The model under review builds one solid part; all positions refer to its coordinate system, in mm. Face numbers are marked on the shaded views. Coordinates: 2 decimals unless noted, no trailing zeros. Order: outer loops, then holes, each group sorted by start corner. A loop starts at its lowest first (then second) coordinate and runs counter-clockwise, first axis right, second up. Notation, with made-up numbers: (12, 87.25) - (26, 87.25) arc R25 cw to (26, 126.25) - close; hole circle Ø6 at (60.5, 69.5). An arc over 180 degrees is marked (long way). Answer in a Markdown table with one row per item.
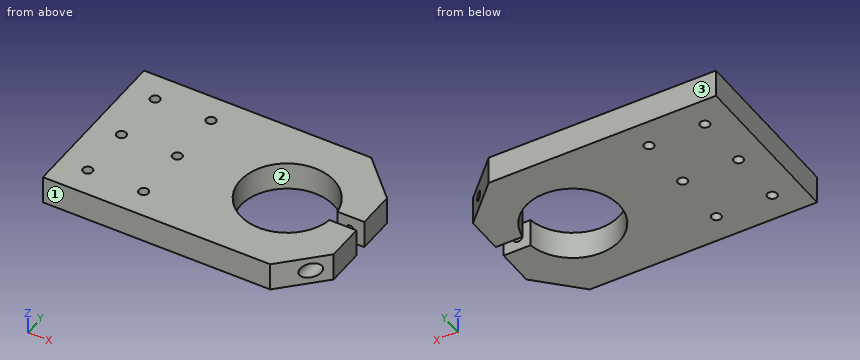
```python
from build123d import *

# Parameters (mm, degrees)
F0_R     = 2.182812
F0_R_2   = 2.182813
F1_DEPTH = 6.35
F2_R     = 3.5
F2_R_2   = 2.182813
F3_DEPTH = 25
F2_R_3   = 1.785938
F4_DEPTH = 35.1
F5_DEPTH = 76.2


with BuildPart() as f1:
    # F0 (on Top) → F1 (new body, symmetric)
    with BuildSketch(Plane.XY):
        with BuildLine():
            ThreePointArc((21.037169, -3), (-21.25, 0), (21.037169, 3))
            Line((21.037169, 3), (33.25, 3))
            Line((33.25, 3), (33.25, 20.1))
            Line((33.25, 20.1), (15.25, 38.1))
            Line((15.25, 38.1), (-88.05, 38.1))
            Line((-88.05, 38.1), (-88.05, -38.1))
            Line((-88.05, -38.1), (15.25, -38.1))
            Line((15.25, -38.1), (33.25, -20.1))
            Line((33.25, -20.1), (33.25, -3))
            Line((33.25, -3), (21.037169, -3))
        make_face()
        with Locations((-75.35, -25.4)):
            Circle(F0_R, mode=Mode.SUBTRACT)
        with Locations((-49.95, -25.4)):
            Circle(F0_R_2, mode=Mode.SUBTRACT)
        with Locations((-75.35, 0)):
            Circle(F0_R, mode=Mode.SUBTRACT)
        with Locations((-49.95, 0)):
            Circle(F0_R_2, mode=Mode.SUBTRACT)
        with Locations((-75.35, 25.4)):
            Circle(F0_R_2, mode=Mode.SUBTRACT)
        with Locations((-49.95, 25.4)):
            Circle(F0_R_2, mode=Mode.SUBTRACT)
    extrude(amount=F1_DEPTH, both=True)

    # F2 (on face) → F3 (cut)
    with BuildSketch(Plane.XZ.offset(38.1)):
        with Locations((26.75, 0)):
            Circle(F2_R)
        with Locations((26.75, 0)):
            Circle(F2_R_2, mode=Mode.SUBTRACT)
    extrude(amount=-F3_DEPTH, mode=Mode.SUBTRACT)

    # F2 (on face) → F4 (cut, through all)
    with BuildSketch(Plane.XZ.offset(38.1)):
        with Locations((26.75, 0)):
            Circle(F2_R_2)
        with Locations((26.75, 0)):
            Circle(F2_R_3, mode=Mode.SUBTRACT)
        with Locations((26.75, 0)):
            Circle(F2_R_3)
    extrude(amount=-F4_DEPTH, mode=Mode.SUBTRACT)

    # F2 (on face) → F5 (cut, through all)
    with BuildSketch(Plane.XZ.offset(38.1)):
        with Locations((26.75, 0)):
            Circle(F2_R_3)
    extrude(amount=-F5_DEPTH, mode=Mode.SUBTRACT)


solid = f1.part
```
Item 1: To check wall thickness, follow line 1 (Y direction, x = -49.95, z = 2.25); line 2 (X direction, y = 6, z = 0.75); line 3 (X direction, y = 25, z = 4.5). State the ranges of each line that lie inside material, in increasing order. Write a range as from..to.
Check values:
| item | result |
|---|---|
| line 1 | -38.1..-27.58, -23.22..-2.18, 2.18..23.22, 27.58..38.1 |
| line 2 | -88.05..-20.39, 20.39..25.13, 28.37..33.25 |
| line 3 | -88.05..-77.5, -73.2..-52.1, -47.8..28.35 |
Item 2: We need section A-A, the plane x = 0. Write out the cut boundary in (y, z), then the cut area to 3 significant figures.
Check values:
| item | result |
|---|---|
| outline | (-38.1, -6.35) - (-21.25, -6.35) - (-21.25, 6.35) - (-38.1, 6.35) - close; (21.25, -6.35) - (38.1, -6.35) - (38.1, 6.35) - (21.25, 6.35) - close |
| area | 428 mm^2 |
Item 3: Clearance check with flat-ended pins moving along their axes: pin 1 Ø3.5 at (x, z) = (26.5, -0.5) entering from -Y; pin 2 Ø1.5 at (y, z) = (21.5, -0.5) entering from +X; pin 3 Ø3.5 at (x, z) = (30, -2.5) entering from -Y. State where each tip first meets the part, or that it passes through.
Check values:
| item | result |
|---|---|
| pin 1 | y = -13.1 |
| pin 2 | x = 32.6 |
| pin 3 | y = -24.99 |
Item 4: We need section C-C, the plane x = -49.95. Write out the cut boundary in (y, z), then the cut area to 3 significant figures.
Check values:
| item | result |
|---|---|
| outline | (-38.1, -6.35) - (-27.58, -6.35) - (-27.58, 6.35) - (-38.1, 6.35) - close; (-23.22, -6.35) - (-2.18, -6.35) - (-2.18, 6.35) - (-23.22, 6.35) - close; (2.18, -6.35) - (23.22, -6.35) - (23.22, 6.35) - (2.18, 6.35) - close; (27.58, -6.35) - (38.1, -6.35) - (38.1, 6.35) - (27.58, 6.35) - close |
| area | 801 mm^2 |
Item 5: We need section D-D, the plane y = 0. Write out the cut boundary in (x, z).
Check values:
| item | result |
|---|---|
| outline | (-88.05, -6.35) - (-77.53, -6.35) - (-77.53, 6.35) - (-88.05, 6.35) - close; (-73.17, -6.35) - (-52.13, -6.35) - (-52.13, 6.35) - (-73.17, 6.35) - close; (-47.77, -6.35) - (-21.25, -6.35) - (-21.25, 6.35) - (-47.77, 6.35) - close |
Item 6: Mouldability with a two-part tool opening along Y and no side actions: class the marked faces 1, 2 and 3 as +Y half, -Y half, draft (parallel to the pull), parting line (faces both ways), or undercut.
Check values:
| item | result |
|---|---|
| face 1 | -Y half |
| face 2 | undercut |
| face 3 | +Y half |
Item 7: We need section B-B, the plane y = -9. Write out the cut boundary in (x, z).
Check values:
| item | result |
|---|---|
| outline | (-88.05, -6.35) - (-19.25, -6.35) - (-19.25, 6.35) - (-88.05, 6.35) - close; (19.25, -6.35) - (33.25, -6.35) - (33.25, 6.35) - (19.25, 6.35) - close; hole circle Ø4.37 at (26.75, 0) |
